```python
from build123d import *

# Parameters (mm, degrees)
BOSS_EXTRUDE1_DEPTH = 6
SKETCH2_R           = 1.25
CUT_EXTRUDE1_DEPTH  = 12
FILLET1_R           = 0.25


with BuildPart() as part:
    # Sketch1 → Boss-Extrude1 (new, symmetric)
    with BuildSketch(Plane(origin=(0, 0, 0), x_dir=(1, 0, 0), z_dir=(0, 1, 0))):
        Polygon((-2.886751346, 0), (-1.443375673, -2.5), (1.443375673, -2.5), (2.886751346, 0), (1.443375673, 2.5), (-1.443375673, 2.5), align=None)
    extrude(amount=BOSS_EXTRUDE1_DEPTH, both=True)

    # Sketch2 → Cut-Extrude1 (cut)
    with BuildSketch(Plane(origin=(0, 6, 0), x_dir=(1, 0, 0), z_dir=(0, 1, 0))):
        with Locations(Location((0, 0, 0), (0, 0, 270))):
            Circle(SKETCH2_R)
    extrude(amount=-CUT_EXTRUDE1_DEPTH, mode=Mode.SUBTRACT)

    # Sketch3 → Cut-Revolve1 (revolve, cut)
    with BuildSketch(Plane.XY):
        with BuildLine():
            Line((2.511751346, 6), (2.886751346, 6))
            Line((2.886751346, 6), (2.886751346, 5.625))
            ThreePointArc((2.886751346, 5.625), (2.776916389, 5.890165043), (2.511751346, 6))
        make_face()
        with BuildLine():
            Line((2.886751346, -6), (2.886751346, -5.625))
            ThreePointArc((2.886751346, -5.625), (2.776916389, -5.890165043), (2.511751346, -6))
            Line((2.511751346, -6), (2.886751346, -6))
        make_face()
    revolve(axis=Axis((0, 5.721589011, 0), (0, -1, 0)), mode=Mode.SUBTRACT)

    # Fillet1
    fillet1_edges = [part.edges().sort_by_distance(p)[0] for p in [
        (0, 6, -1.25),
        (0, -6, -1.25),
    ]]
    fillet(fillet1_edges, radius=FILLET1_R)


solid = part.part
```
The model under review builds one solid part; all positions refer to its coordinate system, in mm. Coordinates: 2 decimals unless noted, no trailing zeros. Write each loop counter-clockwise with the first axis right and the second up, starting at its lowest first coordinate (ties: lowest second). Pieces come first, ordered by that corner, then holes. Notation, with made-up numbers: (70.5, 39) - (117.5, 39) arc R20 ccw to (117.5, 48) - close; hole circle Ø2 at (15.5, -10). An arc over 180 degrees is marked (long way). Answer in a Markdown table with one row per item. Add a question column.
Q1. Consider section B-B on y = -1.5. Give the boundary of the cut face in (x, z).
Q2. Draft analysis for pull direction Z (two halves, no side actions). For faces 1 (the face through (2.175, 0.084, -1.233)), 2 (the face through (2.155, 0.084, 1.268)), 3 (the face through (2, -6, 0)), 4 (the face through (-1.22, 0.08, -0.27)), state which applies: +Z half, -Z half, draft (parallel to the pull), parting line (faces both ways), or undercut.
Q3. To check wall thickness, follow line 1 along Z through (x, y) = (0.05, -4.5); line 2 along Z through (x, y) = (0.7, -4.5); line 3 along X through (y, z) = (1.25, -0.35). State the ranges of each line that lie inside material, in increasing order. Write a range as from..to.
Q4. Consider section A-A on x = 0. Give the boundary of the cut face in (y, z), then the cut area to 3 significant figures.
Q5. Clearance check with flat-ended pins moving along their axes: pin 1 (1.5 mm diameter, centred on y = 3.5, z = 1, fed in from -X); pin 2 (2 mm diameter, centred on x = 0, z = 0, fed in from -Y). State where each tip first meets the part, or that it passes through.
Answers below:
| question | item | result |
|---|---|---|
| 1 | outline | (-2.89, 0) - (-1.44, -2.5) - (1.44, -2.5) - (2.89, 0) - (1.44, 2.5) - (-1.44, 2.5) - close; hole circle Ø2.5 at (0, 0) |
| 2 | face 1 | -Z half |
| 2 | face 2 | +Z half |
| 2 | face 3 | draft |
| 2 | face 4 | undercut |
| 3 | line 1 | -2.5..-1.25, 1.25..2.5 |
| 3 | line 2 | -2.5..-1.04, 1.04..2.5 |
| 3 | line 3 | -2.68..-1.2, 1.2..2.68 |
| 4 | outline | (-6, -2.5) - (6, -2.5) - (6, -1.5) arc R0.25 ccw to (5.75, -1.25) - (-5.75, -1.25) arc R0.25 ccw to (-6, -1.5) - close; (-6, 1.5) arc R0.25 ccw to (-5.75, 1.25) - (5.75, 1.25) arc R0.25 ccw to (6, 1.5) - (6, 2.5) - (-6, 2.5) - close |
| 4 | area | 29.9 mm² |
| 5 | pin 1 | x = -2.74 |
| 5 | pin 2 | through |
